Work out the finished part from the listing and answer in its coordinate system (mm). A direction names the side the tool comes from. Give positions to 0.01 mm unless a question says otherwise; leave off trailing zeros. Order: outer loops, then holes, each group sorted by start corner. A loop starts at its lowest first (then second) coordinate and runs counter-clockwise, first axis right, second up. Notation, with made-up numbers: M 17.5,53.5 L 64.5,53.5 A25 cw 64.5,92.5 Z; hole C -36,10.25 d6. An arc over 180 degrees is marked long. One line per item, written item: value.
from build123d import *

# Parameters (mm, degrees)
SKETCH1_W           = 55
SKETCH1_H           = 45
BOSS_EXTRUDE1_DEPTH = 5
SKETCH3_W           = 55
SKETCH3_H           = 13
BOSS_EXTRUDE5_DEPTH = 20
CHAMFER1_SIZE       = 8
SKETCH5_R           = 4.5
CUT_EXTRUDE2_DEPTH  = 8
BOSS_EXTRUDE7_DEPTH = 48
CUT_EXTRUDE3_DEPTH  = 71.205777697
CHAMFER2_SIZE       = 3.5
CHAMFER3_SIZE       = 3.5
CHAMFER4_SIZE       = 7


with BuildPart() as part:
    # Sketch1 → Boss-Extrude1 (new body)
    with BuildSketch(Plane.XY):
        with Locations((17.145774036, 16.279520652)):
            Rectangle(SKETCH1_W, SKETCH1_H)
    extrude(amount=BOSS_EXTRUDE1_DEPTH)

    # Sketch3 → Boss-Extrude5 (add)
    with BuildSketch(Plane(origin=(0, 0, 0), x_dir=(-1, 0, 0), z_dir=(0, 0, -1))):
        with Locations((-17.145774036, 0.279520652)):
            Rectangle(SKETCH3_W, SKETCH3_H)
    extrude(amount=BOSS_EXTRUDE5_DEPTH)

    # Chamfer1
    chamfer1_edges = [part.edges().sort_by_distance(p)[0] for p in [
        (17.145774036, -6.220479348, 5),
    ]]
    chamfer(chamfer1_edges, length=CHAMFER1_SIZE)

    # Sketch5 → Cut-Extrude2 (cut)
    with BuildSketch(Plane.XZ.offset(6.220479348)):
        with Locations(Location((-0.354225964, -11, 0), (0, 0, 270))):
            Circle(SKETCH5_R)
        with Locations(Location((34.645774036, -11, 0), (0, 0, 270))):
            Circle(SKETCH5_R)
    extrude(amount=-CUT_EXTRUDE2_DEPTH, mode=Mode.SUBTRACT)

    # Sketch7 → Boss-Extrude7 (add)
    with BuildSketch(Plane.ZY.offset(6.854225964)):
        with BuildLine():
            Line((-8.308177677, 10.21387745), (-12.629175087, 12.000050953))
            ThreePointArc((-12.629175087, 12.000050953), (-15.003318067, 13.416764905), (-16.86901604, 15.457060078))
            Line((-16.86901604, 15.457060078), (-15.17096521, 16.605591044))
            ThreePointArc((-15.17096521, 16.605591044), (-1.55, 20.779520652), (-15.17096521, 24.95345026))
            Line((-15.17096521, 24.95345026), (-16.86901604, 26.101981226))
            ThreePointArc((-16.86901604, 26.101981226), (-15.003318067, 28.142276398), (-12.629175087, 29.55899035))
            Line((-12.629175087, 29.55899035), (0, 34.779520652))
            Line((0, 34.779520652), (0, 6.779520652))
            Line((0, 6.779520652), (-8.576470695, 6.779520652))
            ThreePointArc((-8.576470695, 6.779520652), (-7.194534972, 8.39922137), (-8.308177677, 10.21387745))
        make_face()
    extrude(amount=-BOSS_EXTRUDE7_DEPTH)

    # Sketch8 → Cut-Extrude3 (cut, through all)
    with BuildSketch(Plane.ZY.offset(10.354225964)):
        Polygon((0, 34.779520652), (5, 36.846373896), (5, 38.779520652), (0, 38.779520652), align=None)
    extrude(amount=-CUT_EXTRUDE3_DEPTH, mode=Mode.SUBTRACT)

    # Chamfer2
    chamfer2_edges = [part.edges().sort_by_distance(p)[0] for p in [
        (-10.354225964, 6.779520652, -10),
        (-10.354225964, 20.779520652, 0),
    ]]
    chamfer(chamfer2_edges, length=CHAMFER2_SIZE - 0.0001)  # a hair under: the kernel refuses the full size

    # Chamfer3
    chamfer3_edges = [part.edges().sort_by_distance(p)[0] for p in [
        (44.645774036, 20.779520652, 0),
        (44.645774036, 6.779520652, -10),
    ]]
    chamfer(chamfer3_edges, length=CHAMFER3_SIZE - 0.0001)  # a hair under: the kernel refuses the full size

    # Chamfer4
    chamfer4_edges = [part.edges().sort_by_distance(p)[0] for p in [
        (44.645774036, -1.470429348, -20),
        (-10.354225964, -1.470429348, -20),
    ]]
    chamfer(chamfer4_edges, length=CHAMFER4_SIZE)


solid = part.part
(1) Given P1, Ø4, axis at x = 30.5, z = 0, coming from the -Y side; P2, Ø1, axis at x = 10, z = -9, coming from the +Y side; P3, Ø4, axis at x = 5.5, z = -9, coming from the +Y side, each flat-ended and moving along its own axis, determine where each tip first touches the part or whether it passes through.
Findings:
P1: stops at y = -5.22
P2: stops at y = 31.27
P3: stops at y = 31.89
(2) Which of the six approach directions +Z, -Z, +X, -X, +Y, -Y give full straight-line access (tool end or side, diameter ignored) to faces 1 (the flat face through (16.76, -2.16, 1.06)), 2 (the flat face through (41.146, 21, -1)), 3 (the flat face through (16.81, 11.094, -10.438)), 4 (the cylindrical face through (38.44, -2.28, -13.42)), 5 (the flat face through (-6.854, 21, -1))?
Findings:
face 1: +Z, +X, -X, -Y
face 2: -Z, +X, +Y
face 3: -Z, +X, -X
face 4: -Y
face 5: -Z, -X, +Y
(3) Section A-A, the plane z = -9.25 is taken. Give the vertices of the cut face in (x, y), then the cut area to 3 significant figures.
Findings:
outline: M -10.35,-6.22 L -4.5,-6.22 L -4.5,1.78 L 3.79,1.78 L 3.79,-6.22 L 30.5,-6.22 L 30.5,1.78 L 38.79,1.78 L 38.79,-6.22 L 44.65,-6.22 L 44.65,3.28 L 41.15,6.78 L -6.85,6.78 L -10.35,3.28 Z; M -6.85,10.6 L 41.15,10.6 L 41.15,13.33 L -6.85,13.33 Z; M -6.85,28.23 L 41.15,28.23 L 41.15,30.96 L -6.85,30.96 Z
area: 832 mm^2
(4) Section C-C, the plane x = 38.5 is taken. Give the vertices of the cut face in (y, z).
Findings:
outline: M -6.22,-19.15 L 6.78,-19.15 L 6.78,-8.58 A1.81 cw 10.21,-8.31 L 12,-12.63 A9.5 ccw 15.46,-16.87 L 16.61,-15.17 A7.45 cw long 24.95,-15.17 L 26.1,-16.87 A9.5 ccw 29.56,-12.63 L 36.85,5 L 1.78,5 L -6.22,-3 L -6.22,-8.68 L 1.78,-8.68 L 1.78,-13.32 L -6.22,-13.32 Z
(5) Determine the mould class of faces 6 (the flat face through (16.81, 25.52, -16.01)), 7 (the cylindrical face through (1, -2.28, -15.29)), 8 (the flat face through (-8.58, 19.522, 1.725)) for opening direction X: pulls with the +X half, pulls with the -X half, needs draft (parallel to the pull), parting line crosses it, or undercut.
Findings:
face 6: needs draft
face 7: undercut
face 8: pulls with the -X half
(6) Find the intervals of material crossed by probe 1 along X at (y, z) = (-1.5, -11); probe 2 along Y at (x, z) = (18, -9); probe 3 along Y at (x, z) = (17, -12.5), in increasing order. Write a range as from..to.
Findings:
probe 1: x = -10.35..-4.85, 4.15..30.15, 39.15..44.65
probe 2: y = -6.22..6.78, 10.5..13.33, 28.23..31.06
probe 3: y = -6.22..6.78, 11.95..14.2, 27.36..29.61
(7) Section B-B, the plane y = 0 is taken. Give the vertices of the cut face in (x, z).
Findings:
outline: M -10.35,-13 L -3.35,-20 L 37.65,-20 L 44.65,-13 L 44.65,3.22 L -10.35,3.22 Z; hole C -0.35,-11 d9; hole C 34.65,-11 d9
